```python
from build123d import *

# Parameters (mm, degrees)
F0_W          = 64
F0_H          = 74
F0_W_2        = 40
F0_H_2        = 50
F1_DEPTH      = 25
F3_DEPTH      = 25
F3_DEPTH_BACK = 25
F5_DEPTH      = 25
F6_R          = 12
F7_R          = 12
F9_DEPTH      = 25
F9_DEPTH_BACK = 25
F11_DEPTH     = 25


with BuildPart() as f1:
    # F0 (on Top) → F1 (new body)
    with BuildSketch(Plane.XY):
        Rectangle(F0_W, F0_H)
        Rectangle(F0_W_2, F0_H_2, mode=Mode.SUBTRACT)
    extrude(amount=F1_DEPTH)

    # F2 (on Right) → F3 (join, two sides)
    with BuildSketch(Plane.YZ) as f3_sk:
        Polygon((-37, 12.5), (-37, 18.5), (-57, 18.5), (-57, 6.5), (-37, 6.5), align=None)
        Polygon((-57, 6.5), (-57, 18.5), (-121.08587988, -18.5), (-115.8897274573, -27.5), align=None)
    extrude(amount=-F3_DEPTH)
    extrude(f3_sk.sketch, amount=F3_DEPTH_BACK)

    # F4 (on face) → F5 (cut)
    with BuildSketch(Plane(origin=(0, -22.260734985, 38.5567240079), x_dir=(1, 0, 0), z_dir=(0, -0.5, 0.8660254038))):
        with BuildLine():
            Line((0, -79.1134480157), (0, -114.1134480157))
            Line((0, -114.1134480157), (10, -114.1134480157))
            Line((10, -114.1134480157), (10, -69.1134480157))
            ThreePointArc((10, -69.1134480157), (7.0710678119, -76.1845158276), (0, -79.1134480157))
        make_face()
        with BuildLine():
            ThreePointArc((10, -69.1134480157), (0, -59.1134480157), (-10, -69.1134480157))
            ThreePointArc((-10, -69.1134480157), (-7.0710678119, -76.1845158276), (0, -79.1134480157))
            ThreePointArc((0, -79.1134480157), (7.0710678119, -76.1845158276), (10, -69.1134480157))
        make_face()
        with BuildLine():
            Line((-10, -69.1134480157), (-10, -114.1134480157))
            Line((-10, -114.1134480157), (0, -114.1134480157))
            Line((0, -114.1134480157), (0, -79.1134480157))
            ThreePointArc((0, -79.1134480157), (-7.0710678119, -76.1845158276), (-10, -69.1134480157))
        make_face()
    extrude(amount=-F5_DEPTH, mode=Mode.SUBTRACT)

    # F6
    f6_edges = [f1.edges().sort_by_distance(p)[0] for p in [
        (-25, -118.487804, -23),
    ]]
    fillet(f6_edges, radius=F6_R)

    # F7
    f7_edges = [f1.edges().sort_by_distance(p)[0] for p in [
        (25, -118.487804, -23),
    ]]
    fillet(f7_edges, radius=F7_R)

    # F8 (on Right) → F9 (join, two sides)
    with BuildSketch(Plane.YZ) as f9_sk:
        Polygon((57, 19), (37, 19), (37, 6), (57, 6), (124.2447130228, 39.2136804718), (119.0829748267, 49.6641815534), align=None)
    extrude(amount=F9_DEPTH)
    extrude(f9_sk.sketch, amount=-F9_DEPTH_BACK)

    # F10 (on face) → F11 (cut)
    with BuildSketch(Plane(origin=(0, 3.634493279, -7.3584274328), x_dir=(1, 0, 0), z_dir=(0, -0.442849073, 0.8965961736))):
        with BuildLine():
            ThreePointArc((19.7, 116.7630763351), (13, 123.4630763351), (6.3, 116.7630763351))
            Line((6.3, 116.7630763351), (19.7, 116.7630763351))
        make_face()
        with BuildLine():
            Line((19.7, 116.7630763351), (6.3, 116.7630763351))
            ThreePointArc((6.3, 116.7630763351), (13, 110.0630763351), (19.7, 116.7630763351))
        make_face()
        with BuildLine():
            ThreePointArc((-6.3, 116.7630763351), (-13, 123.4630763351), (-19.7, 116.7630763351))
            Line((-19.7, 116.7630763351), (-6.3, 116.7630763351))
        make_face()
        with BuildLine():
            Line((-6.3, 116.7630763351), (-19.7, 116.7630763351))
            ThreePointArc((-19.7, 116.7630763351), (-13, 110.0630763351), (-6.3, 116.7630763351))
        make_face()
        with BuildLine():
            ThreePointArc((19.7, 80.7630763351), (13, 87.4630763351), (6.3, 80.7630763351))
            Line((6.3, 80.7630763351), (19.7, 80.7630763351))
        make_face()
        with BuildLine():
            Line((19.7, 80.7630763351), (6.3, 80.7630763351))
            ThreePointArc((6.3, 80.7630763351), (13, 74.0630763351), (19.7, 80.7630763351))
        make_face()
        with BuildLine():
            ThreePointArc((-6.3, 80.7630763351), (-13, 87.4630763351), (-19.7, 80.7630763351))
            Line((-19.7, 80.7630763351), (-6.3, 80.7630763351))
        make_face()
        with BuildLine():
            Line((-6.3, 80.7630763351), (-19.7, 80.7630763351))
            ThreePointArc((-19.7, 80.7630763351), (-13, 74.0630763351), (-6.3, 80.7630763351))
        make_face()
    extrude(amount=-F11_DEPTH, mode=Mode.SUBTRACT)


solid = f1.part
```
Build history of the part. All positions in model axes, mm. A direction names the side the tool comes from. Give positions to 0.01 mm unless a question says otherwise; leave off trailing zeros. Loops run counter-clockwise (first coordinate to the right, second up) from the corner with the lowest first, then second, coordinate; pieces in that order, holes last.
Item 1: Slice it at C-C, the plane x = -1. List the corners of the cut face in (y, z).
Answers follow:
outline: (-73.5, 8.97) - (-68.3, -0.03) - (-57, 6.5) - (-37, 6.5) - (-37, 0) - (-25, 0) - (-25, 25) - (-37, 25) - (-37, 18.5) - (-57, 18.5) - close; (25, 0) - (37, 0) - (37, 6) - (57, 6) - (124.24, 39.21) - (119.08, 49.66) - (57, 19) - (37, 19) - (37, 25) - (25, 25) - close
Item 2: Which spindle directions (+Z, -Z, +X, -X, +Y, -Y) get a long thin tool onto all of the face, cutting with end or side? Do faces 4 (the face through (-25, 80, 25)), 5 (the face through (0, 47, 6)), 6 (the face through (0.35, 88.48, 34.55)), 7 (the face through (25, -74, 3)), 8 (the face through (0, 25, 12)). Say none if no direction does.
Answers follow:
face 4: +Z, -Z, -X, +Y
face 5: -Z, +X, -X, +Y
face 6: +Z, +X, -X
face 7: +Z, -Z, +X, -Y
face 8: +Z, -Z
Item 3: Slice it at A-A, the plane y = 0. List the corners of the cut face in (x, z).
Answers follow:
outline: (-32, 0) - (-20, 0) - (-20, 25) - (-32, 25) - close; (20, 0) - (32, 0) - (32, 25) - (20, 25) - close
Item 4: Pull direction Y, two halves, no side cores. Call faces 1 (the face through (0.35, 121.7, 44.37)), 2 (the face through (13.872, 72.635, 20.313)), 3 (the face through (-10, -99, -12)): released by +Y, released by -Y, zero draft, split by the parting line, or undercut.
Answers follow:
face 1: released by +Y
face 2: undercut
face 3: zero draft
Item 5: Drill centre lines: line 1 (X direction, y = -20.5, z = 17.5); line 2 (Y direction, x = -8, z = 1); line 3 (Y direction, x = 1.5, z = 24.5). Where is each one in solid material? Low to high.
Answers follow:
line 1: x = -32 to -20, 20 to 32
line 2: y = -73.45 to -66.53, -37 to -25, 25 to 37
line 3: y = -37 to -25, 25 to 37, 68.14 to 94.46
Item 6: Slice it at B-B, the plane z = -8. List the corners of the cut face in (x, y).
Answers follow:
outline: (-25, -102.9) - (-10, -102.9) - (-10, -82.11) - (-25, -82.11) - close; (10, -102.9) - (25, -102.9) - (25, -82.11) - (10, -82.11) - close
Item 7: Flat gauge pins, fed straight in: pin 1 (6 mm diameter, centred on x = 13.5, z = 31, fed in from +Y); pin 2 (12.5 mm diameter, centred on x = -15, z = 9, fed in from -Y); pin 3 (6 mm diameter, centred on x = -8, y = 45.5, fed in from -Z); pin 4 (2 mm diameter, centred on x = -18.5, y = 20, fed in from +Z). Where does each tip first touch, or does it go through?
Answers follow:
pin 1: stops at y = 108.35
pin 2: stops at y = -84.28
pin 3: stops at z = 6
pin 4: passes through
Item 8: Slice it at D-D, the plane y = -46. List the corners of the cut face in (x, z).
Answers follow:
outline: (-25, 6.5) - (25, 6.5) - (25, 18.5) - (-25, 18.5) - close
